Design review of the part shown in the three views and the two pictorial views. Dimensions are in mm from the part's minimum x, y and z. Round coordinates to 2 decimals unless told otherwise and drop trailing zeros. One line per question, with ' | ' between items. Start each with the question number.
Item 1: For L1, parallel to X at y = 9.25, z = 1.3; L2, parallel to Z at x = 7.75, y = 2.75 (1 decimal), list the stretches that pass through material, from the lowest coordinate up. Write a range as [from, to].
Item 2: Add section B-B on z = 1.1. State how many separate pieces and enclosed holes the cut face has, and give its area (3 significant figures).
Item 3: Insertion check: pin 1 Ø1 at (y, z) = (3, 1) entering from -X. The pin has a flat end and moves straight along its axis. Give the tip position at first contact, or say it passes through.
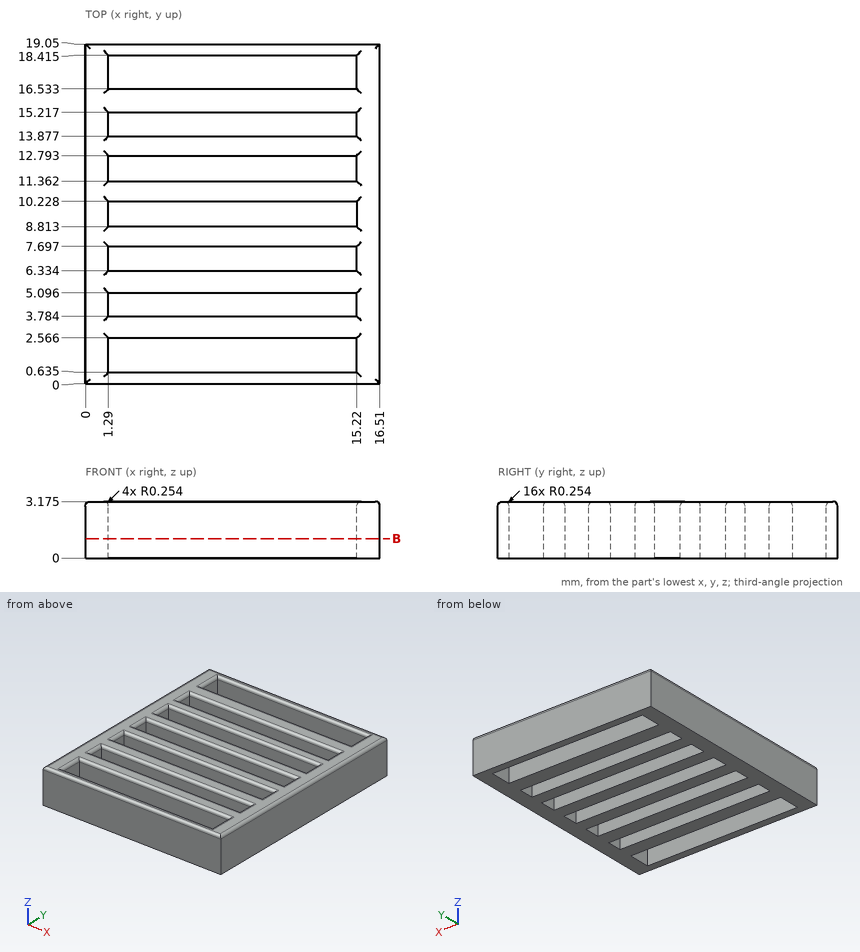
Determined:
1) L1: [0, 1.29], [15.22, 16.51] | L2: [0, 3.2]
2) separate pieces: 1 | enclosed holes: 7 | area: 166 mm2
3) pin 1: x = 0
